Design review of the part built by this model. Coordinates are the model's own, in mm. A direction names the side the tool comes from. Round coordinates to 2 decimals unless told otherwise and drop trailing zeros. Loops run counter-clockwise (first coordinate to the right, second up) from the corner with the lowest first, then second, coordinate; pieces in that order, holes last. Notation, with made-up numbers: (-27.75, 40.25) -> (17.25, 40.25) arc R22 ccw to (17.25, 77.25) -> close; hole circle Ø9 at (-11, 26). An arc over 180 degrees is marked (long way). Answer as CSV lines item,"result". Start each with the question number.
(1) For P1, Ø1.7, axis at x = 11.5, z = 26, coming from the +Y side; P2, Ø2, axis at x = 23, z = 17.5, coming from the +Y side; P3, Ø6, axis at x = 11.5, y = 11, coming from the +Z side, all flat-tipped, find the tip position at first contact; note any pin that passes through.
(2) Draft analysis for pull direction Y (two halves, no side actions). For faces 1 (the face through (15.48, 3.31, 23.595)), 2 (the face through (4.295, 12.215, 29.699)), 3 (the face through (0.95, 6, 15)), state which applies: +Y half, -Y half, draft (parallel to the pull), parting line (faces both ways), or undercut.
(3) Take a section at A-A, the plane z = 15. Write out the cut boundary in (x, y).
(4) To check wall thickness, follow line 1 (Z direction, x = 13, y = 1.75); line 2 (X direction, y = 2.05, z = 25); line 3 (Z direction, x = 10.5, y = 3.5). State the ranges of each line that lie inside material, in increasing order. Write a range as from..to.
(5) Take a section at C-C, the plane y = 2. Write out the cut boundary in (x, z).
(6) Machinability: for faces 4 (the face through (8, 8, 4)), 5 (the face through (12.93, 8.912, 23.796)), 6 (the face through (18.2, 11.99, 0.5)), 7 (the face through (14, 2.55, 7)), which of the approach directions +Z, -Z, +X, -X, +Y, -Y give a long, thin tool a straight path to every point of the face, cutting with its end or side? Answer none if there is none.
Autodesk Fusion 360 part; units mm, degrees
sketch "Sketch1" plane through (0, 0, 0) normal (1, 0, 0) x (0, 0, -1)
  line L0 (0, 12.5) -> (0, 0)
  line L1 (0, 0) -> (-30, 0)
  line L2 (-30, 0) -> (-30, 12.5)
  arc A0 (-22.6, 12.5) -> (-7.4, 12.5) centre (-15, 12.5) ccw
  line L3 (-30, 12.5) -> (-22.6, 12.5)
  line L4 (-7.4, 12.5) -> (0, 12.5)
  dimension "d1" = 15.2
  dimension "d2" = 30
  dimension "d3" = 12.5
extrude "Extrude1" add sketch "Sketch1" along normal blind 26
sketch "Sketch2" plane through (26, 0, 0) normal (1, 0, 0) x (0, 0, -1)
  arc A0 (-22.6, 12.5) -> (-7.4, 12.5) centre (-15, 12.5) ccw
  line L0 (-22.6, 12.5) -> (-30, 12.5)
  line L1 (-30, 12.5) -> (-30, 0)
  line L2 (-30, 0) -> (0, 0)
  line L3 (0, 0) -> (0, 12.5)
  line L4 (0, 12.5) -> (-7.4, 12.5)
  line L5 (-22.6, 12.5) -> (-21, 12.5)
  line L6 (-9, 12.5) -> (-7.4, 12.5)
  arc A1 (-21, 12.5) -> (-9, 12.5) centre (-15, 12.5) ccw
  dimension "d6" = 12
extrude "Extrude2" add sketch "Sketch2" against normal blind 0.95 contours A0 L5 L6 A1
sketch "Sketch3" plane through (0, 6.25, 15) normal (1, 0, 0) x (0, 0, -1)
  line L0 (7.6, 6.25) -> (15, 6.25)
  line L1 (6, 6.25) -> (7.6, 6.25)
  line L2 (-15, 6.25) -> (-7.6, 6.25)
  line L3 (-6, 6.25) -> (-7.6, 6.25)
  arc A0 (-6, 6.25) -> (6, 6.25) centre (0, 6.25) ccw
  arc A1 (-7.6, 6.25) -> (7.6, 6.25) centre (0, 6.25) ccw
  arc A2 (-7.6, 6.25) -> (7.6, 6.25) centre (0, 6.25) ccw
  point P0 (0, 6.25)
  dimension "d9" = 12
extrude "Extrude3" add sketch "Sketch3" along normal blind 0.95
ref_plane "WorkPlane1" through (22, 6.25, 15) normal (1, 0, 0) x (0, 0, -1)
fillet "Fillet1" radius 1 1 edges at (13, 12.5, 0)
fillet "Fillet2" radius 1 1 edges at (13, 12.5, 30)
sketch "Sketch6" plane through (0, 12.5, 0) normal (0, 1, 0) x (-1, 0, 0)
  line L0 (-26, 1) -> (0, 1)
  line L1 (0, 1) -> (0, 9)
  line L2 (0, 9) -> (-0.95, 9)
  line L3 (-0.95, 9) -> (-0.95, 7.4)
  line L4 (-0.95, 7.4) -> (-25.05, 7.4)
  line L5 (-25.05, 7.4) -> (-25.05, 9)
  line L6 (-25.05, 9) -> (-26, 9)
  line L7 (-26, 9) -> (-26, 1)
  circle A0 centre (-13, 5) radius 1.6
  circle A1 centre (-13, 25) radius 1.6
  line L8 (-13, 5) -> (-13, 25) construction
  line L9 (13, 15) -> (-39, 15) construction
  dimension "d15" = 3.2
  dimension "d16" = 3.2
  dimension "d17" = 20
extrude "Extrude4" cut sketch "Sketch6" along normal blind -9 and the other way blind 30 contours A0 | A1
sketch "Sketch7" plane through (22, 6.25, 15) normal (1, 0, 0) x (0, 0, -1)
  arc A0 (-7.6, 6.25) -> (7.6, 6.25) centre (0, 6.25) ccw
  arc A1 (-7.6, 6.25) -> (7.6, 6.25) centre (0, 6.25) ccw
  line L0 (-15, 6.25) -> (-15, -6.25)
  line L1 (-15, -6.25) -> (15, -6.25)
  line L2 (15, -6.25) -> (15, 6.25)
  arc A2 (-10.05, 6.25) -> (10.05, 6.25) centre (0, 6.25) ccw
  line L3 (0, -1.35) -> (0, -3.8) construction
  line L4 (0, -3.8) -> (0, -6.25) construction
  arc A3 (-8.85, 6.2511) -> (8.85, 6.2511) centre (0, 6.2592) ccw
  arc A4 (-8.85, 6.2511) -> (-11.25, 6.2489) centre (-10.05, 6.25) ccw
  arc A5 (-11.25, 6.2489) -> (11.25, 6.2489) centre (0, 6.2592) ccw
  arc A6 (11.25, 6.2489) -> (8.85, 6.2511) centre (10.05, 6.25) ccw
  arc A7 (-10.05, 6.25) -> (10.05, 6.25) centre (0, 6.2592) ccw construction
  dimension "d22" = 1.2
extrude "Extrude5" cut sketch "Sketch7" along normal mid plane 6
ref_plane "WorkPlane2" through (13, 12.5, 15) normal (1, 0, 0) x (0, 0, 1)
mirror "Mirror1" about plane through (13, 12.5, 15) normal (1, 0, 0) of "Extrude5"
ref_plane "WorkPlane3" through (13, 6.25, 15) normal (1, 0, 0) x (0, 0, -1)
sketch "Sketch9" plane through (13, 6.25, 15) normal (1, 0, 0) x (0, 0, -1)
  arc A0 (-6, 6.25) -> (6, 6.25) centre (0, 6.25) ccw
  arc A1 (-6, 6.25) -> (6, 6.25) centre (0, 6.25) ccw
  line L0 (-15, -2) -> (-15, -2.2)
  line L1 (-15, -2.2) -> (-6.7, -2.2)
  line L2 (0, -3.25) -> (0, -2)
  line L3 (-15, 5.25) -> (-15, -6.25)
  line L4 (15, -2) -> (15, -2.2)
  line L5 (15, -2.2) -> (6.7, -2.2)
  line L6 (0, -3.25) -> (0, -2)
  line L7 (-9.5, 6.25) -> (-15, 6.25)
  line L8 (-15, 6.25) -> (-15, -2)
  line L9 (9.5, 6.25) -> (15, 6.25)
  line L10 (15, 6.25) -> (15, -2)
  line L11 (6.7, -0.485) -> (6.7, -2.2)
  line L12 (-6.7, -0.485) -> (-6.7, -2.2)
  arc A2 (-9.5, 6.25) -> (-6.7, -0.485) centre (0, 6.25) ccw
  arc A3 (6.7, -0.485) -> (9.5, 6.25) centre (0, 6.25) ccw
  dimension "d34" = 19
  dimension "d44" = 8.3
  dimension "d45" = 8.3
  dimension "d50" = 0.2
  dimension "d51" = 0.2
extrude "Extrude8" cut sketch "Sketch9" along normal mid plane 10
sketch "Sketch11" plane through (0, 4.05, 0) normal (0, 1, 0) x (-1, 0, 0)
  line L0 (-8, 8.3) -> (-18, 8.3)
  line L1 (-18, 8.3) -> (-18, 0)
  line L2 (-8, 0) -> (-8, 8.3)
  line L3 (-9.7091, 25) -> (-11.3546, 27.85)
  line L4 (-11.3546, 27.85) -> (-14.6454, 27.85)
  line L5 (-14.6454, 27.85) -> (-16.2909, 25)
  line L6 (-16.2909, 25) -> (-14.6454, 22.15)
  line L7 (-14.6454, 22.15) -> (-11.3546, 22.15)
  line L8 (-11.3546, 22.15) -> (-9.7091, 25)
  circle A0 centre (-13, 25) radius 1.6 construction
  point P0 (-13, 25)
  dimension "d38" = 2.85
extrude "Extrude9" cut sketch "Sketch11" against normal blind 1.5
sketch "Sketch12" plane through (0, 4.05, 0) normal (0, 1, 0) x (-1, 0, 0)
  line L0 (-8, 8.3) -> (-18, 8.3)
  line L1 (-18, 8.3) -> (-18, 0)
  line L2 (-18, 0) -> (-8, 0)
  line L3 (-8, 0) -> (-8, 8.3)
  line L4 (-15.85, 3.3546) -> (-13, 1.7091)
  line L5 (-13, 1.7091) -> (-10.15, 3.3546)
  line L6 (-10.15, 3.3546) -> (-10.15, 6.6454)
  line L7 (-10.15, 6.6454) -> (-13, 8.2909)
  line L8 (-13, 8.2909) -> (-15.85, 6.6454)
  line L9 (-15.85, 6.6454) -> (-15.85, 3.3546)
  point P0 (-13, 5)
  dimension "d41" = 2.85
extrude "Extrude10" cut sketch "Sketch12" against normal blind 1.5 contours L4 L5 L6 L7 L8 L9
chamfer "Chamfer1" distance 0.5 angle 45 8 edges at (18, 7.775, 0) (18, 12.2071, 0.2929) (18, 12.5, 3.25) (13, 12.5, 5.5) (8, 12.5, 3.25) (8, 12.2071, 0.2929) (8, 7.775, 0) (13, 4.05, 0)
chamfer "Chamfer2" distance 0.5 angle 45 8 edges at (8, 7.775, 30) (8, 12.2071, 29.7071) (8, 12.5, 26.75) (13, 12.5, 24.5) (18, 12.5, 26.75) (18, 12.2071, 29.7071) (18, 7.775, 30) (13, 4.05, 30)
fillet "Fillet3" radius 2 1 edges at (13, 5.765, 21.7)
fillet "Fillet4" radius 2 1 edges at (13, 5.765, 8.3)
fillet "Fillet5" radius 1 3 edges at (26, 12.5, 25) (26, 12.2071, 29.7071) (26, 5.75, 30)
fillet "Fillet6" radius 1 9 edges at (26, 5.75, 0) (26, 12.2071, 0.2929) (26, 12.5, 5) (0, 12.5, 5) (0, 12.2071, 0.2929) (0, 5.75, 0) (0, 5.75, 30) (0, 12.2071, 29.7071) (0, 12.5, 25)
ref_plane "WorkPlane4" through (13, 5.75, 15) normal (0, 0, 1) x (0, -1, 0)
equation "d10 = wall_width"
equation "wall_width = 0.95 mm"
equation "nut_depth = 3 mm"
The answers:
1,P1,"y = 2.55"
1,P2,"y = 5.75"
1,P3,"z = 24.49"
2,face 1,"undercut"
2,face 2,"+Y half"
2,face 3,"draft"
3,outline,"(0, 0) -> (26, 0) -> (26, 6.5) -> (25.05, 6.5) -> (25.05, 4.9) -> (0.95, 4.9) -> (0.95, 6.5) -> (0, 6.5) -> close; hole (1, 1.26) -> (7, 1.26) -> (7, 3.66) -> (1, 3.66) -> close; hole (19, 1.26) -> (25, 1.26) -> (25, 3.66) -> (19, 3.66) -> close"
4,line 1,"0..3.4, 6.6..23.4, 26.6..30"
4,line 2,"0..11.4, 14.6..26"
4,line 3,"0..3.15, 6.85..23.63, 26.37..30"
5,outline,"(0, 1) arc R1 ccw to (1, 0) -> (25, 0) arc R1 ccw to (26, 1) -> (26, 29) arc R1 ccw to (25, 30) -> (1, 30) arc R1 ccw to (0, 29) -> close; hole (1, 10.99) -> (7, 10.99) -> (7, 19.01) -> (1, 19.01) -> close; hole circle Ø3.2 at (13, 5); hole circle Ø3.2 at (13, 25); hole (19, 10.99) -> (25, 10.99) -> (25, 19.01) -> (19, 19.01) -> close"
6,face 4,"-Z"
6,face 5,"+Z"
6,face 6,"-Z, +Y"
6,face 7,"none"
